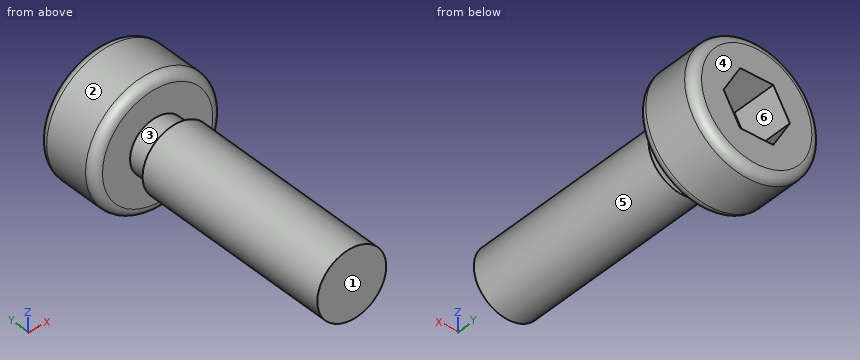
from build123d import *

# Parameters (mm, degrees)
CUT_EXTRUDE_1_DEPTH = 2


with BuildPart() as part:
    # 草图1 → 旋转1 (revolve)
    with BuildSketch(Plane.XY):
        with BuildLine():
            Line((0, 12.8), (-2.4, 12.8))
            ThreePointArc((-2.4, 12.8), (-2.682842712, 12.682842712), (-2.8, 12.4))
            Line((-2.8, 12.4), (-2.8, 10.4))
            ThreePointArc((-2.8, 10.4), (-2.682842712, 10.117157288), (-2.4, 10))
            Line((-2.4, 10), (-1.2, 10))
            Line((-1.2, 10), (-1.2, 9))
            Line((-1.2, 9), (-1.5, 9))
            Line((-1.5, 9), (-1.5, 0))
            Line((-1.5, 0), (0, 0))
            Line((0, 0), (0, 12.8))
        make_face()
    revolve(axis=Axis((0, 0, 0), (0, 1, 0)))

    # 草图2 → 切除-拉伸1 (cut)
    with BuildSketch(Plane(origin=(0, 12.8, 0), x_dir=(1, 0, 0), z_dir=(0, 1, 0))):
        Polygon((-0.721687836, 1.25), (-1.443375673, 0), (-0.721687836, -1.25), (0.721687836, -1.25), (1.443375673, 0), (0.721687836, 1.25), align=None)
    extrude(amount=-CUT_EXTRUDE_1_DEPTH, mode=Mode.SUBTRACT)


solid = part.part
CAD build for the part. Positions are in the model's coordinates, mm. Face numbers are marked on the shaded views. A direction names the side the tool comes from. Round coordinates to 2 decimals unless told otherwise and drop trailing zeros. Write each loop counter-clockwise with the first axis right and the second up, starting at its lowest first coordinate (ties: lowest second). Pieces come first, ordered by that corner, then holes. Notation, with made-up numbers: M -2.5,37 L 50.5,37 A33 cw 50.5,76 Z; hole C 48,77.25 d4. An arc over 180 degrees is marked long. Use a Markdown table: item, result. Add a question column.
1. Flat gauge pins, fed straight in: P1, Ø1.5, axis at y = 1.5, z = -0.5, coming from the -X side; P2, Ø0.8, axis at x = 0, z = -0.5, coming from the +Y side. Where does each tip first touch, or does it go through?
2. 3-axis set-ups, long thin cutter, end or side, ignore diameter. For the marked faces 5 and 6: which of +Z, -Z, +X, -X, +Y, -Y reach the whole face in a straight line?
3. Slice it at A-A on x = 0. Give the cut face in (y, z).
4. Drill centre lines: probe 1 along Y at (x, z) = (-0.05, 0.85); probe 2 along Y at (x, z) = (1.2, 0.85); probe 3 along Z at (x, y) = (0, 9.75). Where is each one in solid material? Low to high.
5. Slice it at B-B on y = 6.5. Give the cut face in (x, z).
6. Pull direction Y, two halves, no side cores. Call the marked faces 1, 2, 3 and 4: released by +Y, released by -Y, zero draft, split by the parting line, or undercut.
Reply:
| question | item | result |
|---|---|---|
| 1 | P1 | stops at x = -1.5 |
| 1 | P2 | stops at y = 10.8 |
| 2 | face 5 | -Y |
| 2 | face 6 | +Y |
| 3 | outline | M 0,-1.5 L 9,-1.5 L 9,-1.2 L 10,-1.2 L 10,-2.4 A0.4 ccw 10.4,-2.8 L 12.4,-2.8 A0.4 ccw 12.8,-2.4 L 12.8,-1.25 L 10.8,-1.25 L 10.8,1.25 L 12.8,1.25 L 12.8,2.4 A0.4 ccw 12.4,2.8 L 10.4,2.8 A0.4 ccw 10,2.4 L 10,1.2 L 9,1.2 L 9,1.5 L 0,1.5 Z |
| 4 | probe 1 | y = 0 to 10.8 |
| 4 | probe 2 | y = 0 to 9, 10 to 12.8 |
| 4 | probe 3 | z = -1.2 to 1.2 |
| 5 | outline | C 0,0 d3 |
| 6 | face 1 | released by -Y |
| 6 | face 2 | zero draft |
| 6 | face 3 | undercut |
| 6 | face 4 | released by +Y |
